Work out the finished part from the listing and answer in its coordinate system (mm). A direction names the side the tool comes from. Coordinates: 2 decimals unless noted, no trailing zeros. Loops run counter-clockwise (first coordinate to the right, second up) from the corner with the lowest first, then second, coordinate; pieces in that order, holes last. Notation, with made-up numbers: (28.25, 23.25) -> (74.25, 23.25) arc R13 cw to (74.25, 45.25) -> close; hole circle Ø4 at (50, -24.5). An arc over 180 degrees is marked (long way). Use a Markdown table: item, result. Add a question column.
```python
from build123d import *

# Parameters (mm, degrees)
SKETCH1_R               = 50
BOSS_EXTRUDE1_DEPTH     = 20
CUT_EXTRUDE4_DEPTH      = 74.484692283
CUT_EXTRUDE4_DEPTH_BACK = 74.484692283
SKETCH3_R               = 46
SKETCH4_R               = 48
CUT_EXTRUDE5_DEPTH      = 8


with BuildPart() as part:
    # Sketch1 → Boss-Extrude1 (new body)
    with BuildSketch(Plane.XY):
        Circle(SKETCH1_R)
    extrude(amount=BOSS_EXTRUDE1_DEPTH)

    # Sketch3 → Cut-Extrude4 (cut, two sides: drawn at the far end of the back side and taken through both)
    with BuildSketch(Plane(origin=(0, 0, 0), x_dir=(-1, 0, 0), z_dir=(0, 0, -1)).offset(-CUT_EXTRUDE4_DEPTH_BACK)):
        Circle(SKETCH3_R)
    extrude(amount=CUT_EXTRUDE4_DEPTH + CUT_EXTRUDE4_DEPTH_BACK, mode=Mode.SUBTRACT)

    # Sketch4 → Cut-Extrude5 (cut, symmetric)
    with BuildSketch(Plane(origin=(0, 0, 10), x_dir=(-1, 0, 0), z_dir=(0, 0, -1))):
        Circle(SKETCH4_R)
    extrude(amount=CUT_EXTRUDE5_DEPTH, both=True, mode=Mode.SUBTRACT)


solid = part.part
```
Item 1: Section C-C (z = 14) is taken. Determine the outline of the cut face in (x, y).
Item 2: Section A-A (y = 0) is taken. Determine the outline of the cut face in (x, z), then the cut area to 3 significant figures.
Item 3: Section B-B (x = -19) is taken. Determine the outline of the cut face in (y, z), then the cut area to 3 significant figures.
Item 4: For a pull along X with two mould halves and no side action, classify faces 3 (the face through (47.69, 15.02, 9.86)), 4 (the face through (5.99, 45.61, 1.01)), 5 (the face through (22, -41, 20)) as +X half, -X half, draft (parallel to the pull), parting line (faces both ways), or undercut.
Item 5: Find the intervals of material crossed by probe 1 along Z at (x, y) = (-25, -40); probe 2 along Y at (x, z) = (0, 11.25); probe 3 along Y at (x, z) = (-21, 15.5), in increasing order.
Item 6: Given pin 1 (2 mm diameter, centred on y = 34, z = 15, fed in from +X); pin 2 (6 mm diameter, centred on x = -33, z = 5, fed in from -Y); pin 3 (8 mm diameter, centred on x = 19.5, z = 7.5, fed in from -Y), each flat-ended and moving along its own axis, determine where each tip first touches the part or whether it passes through.
Item 7: For faces 1 (the face through (47.954, 2.11, 9.888)), 2 (the face through (5.99, 45.61, 19.01)), determine the directions among +Z, -Z, +X, -X, +Y, -Y from which every point of the face is accessible in a straight line to the end or side of a thin tool.
Output:
| question | item | result |
|---|---|---|
| 1 | outline | circle Ø100 at (0, 0); hole circle Ø96 at (0, 0) |
| 2 | outline | (-50, 0) -> (-46, 0) -> (-46, 2) -> (-48, 2) -> (-48, 18) -> (-46, 18) -> (-46, 20) -> (-50, 20) -> close; (46, 0) -> (50, 0) -> (50, 20) -> (46, 20) -> (46, 18) -> (48, 18) -> (48, 2) -> (46, 2) -> close |
| 2 | area | 96.0 mm2 |
| 3 | outline | (-46.25, 0) -> (-41.89, 0) -> (-41.89, 2) -> (-44.08, 2) -> (-44.08, 18) -> (-41.89, 18) -> (-41.89, 20) -> (-46.25, 20) -> close; (41.89, 0) -> (46.25, 0) -> (46.25, 20) -> (41.89, 20) -> (41.89, 18) -> (44.08, 18) -> (44.08, 2) -> (41.89, 2) -> close |
| 3 | area | 104 mm2 |
| 4 | face 3 | parting line |
| 4 | face 4 | undercut |
| 4 | face 5 | draft |
| 5 | probe 1 | z = 0 to 2, 18 to 20 |
| 5 | probe 2 | y = -50 to -48, 48 to 50 |
| 5 | probe 3 | y = -45.38 to -43.16, 43.16 to 45.38 |
| 6 | pin 1 | stops at x = 37.56 |
| 6 | pin 2 | stops at y = -40 |
| 6 | pin 3 | stops at y = -47.54 |
| 7 | face 1 | none |
| 7 | face 2 | +Z, -Z |
